Part model, mm, in its own coordinate system. A direction names the side the tool comes from. Coordinates: 2 decimals unless noted, no trailing zeros. Order: outer loops, then holes, each group sorted by start corner. A loop starts at its lowest first (then second) coordinate and runs counter-clockwise, first axis right, second up.
1) Cut at C-C (y = 13). List the corners of the cut face in (x, z), and give its area (3 significant figures).
2) Tool access for faces 1 (the flat face through (37.5, 11, 30)), 2 (the flat face through (60, 10, 20)), 3 (the flat face through (55, 9, 10)), 4 (the flat face through (0, 10, 20)): list every direction of +Z, -Z, +X, -X, +Y, -Y with a clear straight run to the whole face (end or side of a thin tool).
3) Cut at B-B (z = 30). List the corners of the cut face in (x, y), and give its area (3 significant figures).
4) Pin check, flat tips, straight feed: pin 1 Ø2.5 at (x, z) = (5, 29.5) entering from +Y; pin 2 Ø9 at (y, z) = (12.5, 27.5) entering from +X; pin 3 Ø1 at (x, y) = (38.5, 10.5) entering from -Z. Stop position of each tip, or through.
5) Wall check: L1, parallel to Z at x = 65, y = 2.4; L2, parallel to X at y = 3.45, z = 10; L3, parallel to Z at x = 55, y = 12.5. Give the ranges that are in metal, low to high.
6) Cut at A-A (x = 65). List the corners of the cut face in (y, z).
7) Mould opens along Z. For faces 5 (the cylindrical face through (30, 4, 16)), 6 (the flat face through (21, 12, 20)), 7 (the cylindrical face through (57.217, 12.042, 10.919)) say: +Z half, -Z half, draft (parallel to the pull), parting line (faces both ways), or undercut.
8) Cut at D-D (z = 18.5). List the corners of the cut face in (x, y), and give its area (3 significant figures).
```python
from build123d import *

# Parameters (mm, degrees)
BASE_MORS_DEPTH                    = 40
ESQUISSE2_R                        = 11
EMPLACEMENT_MOTEUR_DEPTH           = 41
ESQUISSE3_R                        = 1.5
TROU_FIXATIONS_BASE_DEPTH          = 6
ESQUISSE4_R                        = 2.4
TROU_FIXATION_MORS_SUPERIEUR_DEPTH = 6
ESQUISSE6_W                        = 3.5
ESQUISSE6_H                        = 12
ENCOCHE_MOTEUR_DEPTH               = 20


with BuildPart() as part:
    # Esquisse1 → base_mors (new body)
    with BuildSketch(Plane.XY):
        Polygon((60, 15), (60, 5), (70, 5), (70, 0), (60, 0), (0, 0), (-10, 0), (-10, 5), (0, 5), (0, 15), align=None)
    extrude(amount=BASE_MORS_DEPTH)

    # Esquisse2 → emplacement_moteur (cut, through all)
    with BuildSketch(Plane.XY.offset(40)):
        with Locations((30, 15)):
            Circle(ESQUISSE2_R)
    extrude(amount=-EMPLACEMENT_MOTEUR_DEPTH, mode=Mode.SUBTRACT)

    # Esquisse3 → trou_fixations_base (cut, through all)
    with BuildSketch(Plane(origin=(0, 5, 0), x_dir=(1, 0, 0), z_dir=(0, 1, 0))):
        with Locations((-5, -10)):
            Circle(ESQUISSE3_R)
        with Locations((65, -10)):
            Circle(ESQUISSE3_R)
        with Locations((65, -30)):
            Circle(ESQUISSE3_R)
        with Locations((-5, -30)):
            Circle(ESQUISSE3_R)
    extrude(amount=-TROU_FIXATIONS_BASE_DEPTH, mode=Mode.SUBTRACT)

    # Esquisse4 → trou_fixation_mors_superieur (cut)
    with BuildSketch(Plane(origin=(0, 15, 0), x_dir=(1, 0, 0), z_dir=(0, 1, 0))):
        with Locations((5, -10)):
            Circle(ESQUISSE4_R)
        with Locations((55, -10)):
            Circle(ESQUISSE4_R)
        with Locations((55, -30)):
            Circle(ESQUISSE4_R)
        with Locations((5, -30)):
            Circle(ESQUISSE4_R)
    extrude(amount=-TROU_FIXATION_MORS_SUPERIEUR_DEPTH, mode=Mode.SUBTRACT)

    # Esquisse6 → encoche moteur (add)
    with BuildSketch(Plane.XY.offset(40)):
        with Locations((20.75, 9)):
            Rectangle(ESQUISSE6_W, ESQUISSE6_H)
        with Locations((39.25, 9)):
            Rectangle(ESQUISSE6_W, ESQUISSE6_H)
    extrude(amount=-ENCOCHE_MOTEUR_DEPTH)


solid = part.part
```
Geometry check:
1. outline: (0, 0) - (19.18, 0) - (19.18, 20) - (22.5, 20) - (22.5, 40) - (0, 40) - close; (37.5, 20) - (40.82, 20) - (40.82, 0) - (60, 0) - (60, 40) - (37.5, 40) - close; hole circle Ø4.8 at (5, 10); hole circle Ø4.8 at (5, 30); hole circle Ø4.8 at (55, 10); hole circle Ø4.8 at (55, 30)
1. area: 1,590 mm2
2. face 1: +Z, -Z, +Y
2. face 2: +Z, -Z, +X, +Y
2. face 3: +Y
2. face 4: +Z, -Z, -X, +Y
3. outline: (-10, 0) - (-6.5, 0) - (-6.5, 5) - (-10, 5) - close; (-3.5, 0) - (63.5, 0) - (63.5, 5) - (60, 5) - (60, 15) - (57.4, 15) - (57.4, 9) - (52.6, 9) - (52.6, 15) - (37.5, 15) - (37.5, 6.95) arc R11 cw to (22.5, 6.95) - (22.5, 15) - (7.4, 15) - (7.4, 9) - (2.6, 9) - (2.6, 15) - (0, 15) - (0, 5) - (-3.5, 5) - close; (66.5, 0) - (70, 0) - (70, 5) - (66.5, 5) - close
3. area: 761 mm2
4. pin 1: stops at y = 9
4. pin 2: stops at x = 60
4. pin 3: stops at z = 20
5. L1: z = 0 to 8.5, 11.5 to 28.5, 31.5 to 40
5. L2: x = -10 to -6.5, -3.5 to 63.5, 66.5 to 70
5. L3: z = 0 to 7.6, 12.4 to 27.6, 32.4 to 40
6. outline: (0, 0) - (5, 0) - (5, 8.5) - (0, 8.5) - close; (0, 11.5) - (5, 11.5) - (5, 28.5) - (0, 28.5) - close; (0, 31.5) - (5, 31.5) - (5, 40) - (0, 40) - close
7. face 5: draft
7. face 6: -Z half
7. face 7: undercut
8. outline: (-10, 0) - (70, 0) - (70, 5) - (60, 5) - (60, 15) - (41, 15) arc R11 cw to (19, 15) - (0, 15) - (0, 5) - (-10, 5) - close
8. area: 810 mm2
